from build123d import *

# Parameters (mm, degrees)
SKETCH2_R          = 32.5
CUT_EXTRUDE1_DEPTH = 3
SKETCH3_R          = 1.25
CUT_EXTRUDE2_DEPTH = 12
CUT_EXTRUDE3_REACH = 44.5
SKETCH4_R          = 1.25
SKETCH4_R_2        = 2.1
CHAMFER1_SIZE      = 0.5
CHAMFER2_SIZE      = 0.5


with BuildPart() as part:
    # Sketch1 → Revolve1 (revolve)
    with BuildSketch(Plane.YX):
        Polygon((-32.5, -4.5), (-32.5, -0.5), (-25, -0.5), (-25, 0), (-22.5, 0), (-22.5, 7), (-14, 7), (-14, 10.5), (-10.5, 10.5), (-10.5, 38), (-8.5, 38), (-8.5, 30), (0, 30), (0, 9.5), (-8, 9.5), (-8, 4.5), (-20, 4.5), (-20, -7.5), (-24, -7.5), (-24, -4.5), align=None)
    revolve(axis=Axis((0, 0, 0), (1, 0, 0)))

    # Sketch2 → Cut-Extrude1 (cut)
    with BuildSketch(Plane.ZY.offset(7.5)):
        Circle(SKETCH2_R)
        with BuildLine():
            Line((-8.94427191, 22), (8.94427191, 22))
            ThreePointArc((8.94427191, 22), (9.598925581, 21.927700219), (10.22202504, 21.714285714))
            ThreePointArc((10.22202504, 21.714285714), (16.970562748, 16.970562748), (21.714285714, 10.22202504))
            ThreePointArc((21.714285714, 10.22202504), (21.927700219, 9.598925581), (22, 8.94427191))
            Line((22, 8.94427191), (22, -8.94427191))
            ThreePointArc((22, -8.94427191), (21.927700219, -9.598925581), (21.714285714, -10.22202504))
            ThreePointArc((21.714285714, -10.22202504), (16.970562748, -16.970562748), (10.22202504, -21.714285714))
            ThreePointArc((10.22202504, -21.714285714), (9.598925581, -21.927700219), (8.94427191, -22))
            Line((8.94427191, -22), (-8.94427191, -22))
            ThreePointArc((-8.94427191, -22), (-9.598925581, -21.927700219), (-10.22202504, -21.714285714))
            ThreePointArc((-10.22202504, -21.714285714), (-16.970562748, -16.970562748), (-21.714285714, -10.22202504))
            ThreePointArc((-21.714285714, -10.22202504), (-21.927700219, -9.598925581), (-22, -8.94427191))
            Line((-22, -8.94427191), (-22, 8.94427191))
            ThreePointArc((-22, 8.94427191), (-21.927700219, 9.598925581), (-21.714285714, 10.22202504))
            ThreePointArc((-21.714285714, 10.22202504), (-16.970562748, 16.970562748), (-10.22202504, 21.714285714))
            ThreePointArc((-10.22202504, 21.714285714), (-9.598925581, 21.927700219), (-8.94427191, 22))
        make_face(mode=Mode.SUBTRACT)
    extrude(amount=-CUT_EXTRUDE1_DEPTH, mode=Mode.SUBTRACT)

    # Sketch3 → Cut-Extrude2 (cut)
    with BuildSketch(Plane(origin=(30, 0, 0), x_dir=(0, 0, -1), z_dir=(1, 0, 0))):
        with Locations((0, 6)):
            Circle(SKETCH3_R)
        with Locations((5.706339098, 1.854101966)):
            Circle(SKETCH3_R)
        with Locations((3.526711514, -4.854101966)):
            Circle(SKETCH3_R)
        with Locations((-3.526711514, -4.854101966)):
            Circle(SKETCH3_R)
        with Locations((-5.706339098, 1.854101966)):
            Circle(SKETCH3_R)
    extrude(amount=-CUT_EXTRUDE2_DEPTH, mode=Mode.SUBTRACT)

    # Sketch4 → Cut-Extrude3 (cut, up to next)
    with BuildSketch(Plane.ZY.offset(4.5), mode=Mode.PRIVATE) as cut_extrude3_sk1:
        with Locations((0, 27)):
            Circle(SKETCH4_R)
    cut_extrude3_tool1 = extrude(cut_extrude3_sk1.sketch, amount=-CUT_EXTRUDE3_REACH, mode=Mode.PRIVATE) & part.part
    add(cut_extrude3_tool1.solids().sort_by_distance((-4.5, 27, 0))[0], mode=Mode.SUBTRACT)
    # Sketch4 → Cut-Extrude3 (cut, up to next)
    with BuildSketch(Plane.ZY.offset(4.5), mode=Mode.PRIVATE) as cut_extrude3_sk2:
        with Locations((10.906477822, 26.330566677)):
            Circle(SKETCH4_R_2)
    cut_extrude3_tool2 = extrude(cut_extrude3_sk2.sketch, amount=-CUT_EXTRUDE3_REACH, mode=Mode.PRIVATE) & part.part
    add(cut_extrude3_tool2.solids().sort_by_distance((-4.5, 26.330567, 10.906478))[0], mode=Mode.SUBTRACT)
    # Sketch4 → Cut-Extrude3 (cut, up to next)
    with BuildSketch(Plane.ZY.offset(4.5), mode=Mode.PRIVATE) as cut_extrude3_sk3:
        with Locations((19.091883092, 19.091883092)):
            Circle(SKETCH4_R)
    cut_extrude3_tool3 = extrude(cut_extrude3_sk3.sketch, amount=-CUT_EXTRUDE3_REACH, mode=Mode.PRIVATE) & part.part
    add(cut_extrude3_tool3.solids().sort_by_distance((-4.5, 19.091883, 19.091883))[0], mode=Mode.SUBTRACT)
    # Sketch4 → Cut-Extrude3 (cut, up to next)
    with BuildSketch(Plane.ZY.offset(4.5), mode=Mode.PRIVATE) as cut_extrude3_sk4:
        with Locations((26.330566677, 10.906477822)):
            Circle(SKETCH4_R_2)
    cut_extrude3_tool4 = extrude(cut_extrude3_sk4.sketch, amount=-CUT_EXTRUDE3_REACH, mode=Mode.PRIVATE) & part.part
    add(cut_extrude3_tool4.solids().sort_by_distance((-4.5, 10.906478, 26.330567))[0], mode=Mode.SUBTRACT)
    # Sketch4 → Cut-Extrude3 (cut, up to next)
    with BuildSketch(Plane.ZY.offset(4.5), mode=Mode.PRIVATE) as cut_extrude3_sk5:
        with Locations((27, 0)):
            Circle(SKETCH4_R)
    cut_extrude3_tool5 = extrude(cut_extrude3_sk5.sketch, amount=-CUT_EXTRUDE3_REACH, mode=Mode.PRIVATE) & part.part
    add(cut_extrude3_tool5.solids().sort_by_distance((-4.5, 0, 27))[0], mode=Mode.SUBTRACT)
    # Sketch4 → Cut-Extrude3 (cut, up to next)
    with BuildSketch(Plane.ZY.offset(4.5), mode=Mode.PRIVATE) as cut_extrude3_sk6:
        with Locations((26.330566677, -10.906477822)):
            Circle(SKETCH4_R_2)
    cut_extrude3_tool6 = extrude(cut_extrude3_sk6.sketch, amount=-CUT_EXTRUDE3_REACH, mode=Mode.PRIVATE) & part.part
    add(cut_extrude3_tool6.solids().sort_by_distance((-4.5, -10.906478, 26.330567))[0], mode=Mode.SUBTRACT)
    # Sketch4 → Cut-Extrude3 (cut, up to next)
    with BuildSketch(Plane.ZY.offset(4.5), mode=Mode.PRIVATE) as cut_extrude3_sk7:
        with Locations((19.091883092, -19.091883092)):
            Circle(SKETCH4_R)
    cut_extrude3_tool7 = extrude(cut_extrude3_sk7.sketch, amount=-CUT_EXTRUDE3_REACH, mode=Mode.PRIVATE) & part.part
    add(cut_extrude3_tool7.solids().sort_by_distance((-4.5, -19.091883, 19.091883))[0], mode=Mode.SUBTRACT)
    # Sketch4 → Cut-Extrude3 (cut, up to next)
    with BuildSketch(Plane.ZY.offset(4.5), mode=Mode.PRIVATE) as cut_extrude3_sk8:
        with Locations((10.906477822, -26.330566677)):
            Circle(SKETCH4_R_2)
    cut_extrude3_tool8 = extrude(cut_extrude3_sk8.sketch, amount=-CUT_EXTRUDE3_REACH, mode=Mode.PRIVATE) & part.part
    add(cut_extrude3_tool8.solids().sort_by_distance((-4.5, -26.330567, 10.906478))[0], mode=Mode.SUBTRACT)
    # Sketch4 → Cut-Extrude3 (cut, up to next)
    with BuildSketch(Plane.ZY.offset(4.5), mode=Mode.PRIVATE) as cut_extrude3_sk9:
        with Locations((0, -27)):
            Circle(SKETCH4_R)
    cut_extrude3_tool9 = extrude(cut_extrude3_sk9.sketch, amount=-CUT_EXTRUDE3_REACH, mode=Mode.PRIVATE) & part.part
    add(cut_extrude3_tool9.solids().sort_by_distance((-4.5, -27, 0))[0], mode=Mode.SUBTRACT)
    # Sketch4 → Cut-Extrude3 (cut, up to next)
    with BuildSketch(Plane.ZY.offset(4.5), mode=Mode.PRIVATE) as cut_extrude3_sk10:
        with Locations((-10.906477822, -26.330566677)):
            Circle(SKETCH4_R_2)
    cut_extrude3_tool10 = extrude(cut_extrude3_sk10.sketch, amount=-CUT_EXTRUDE3_REACH, mode=Mode.PRIVATE) & part.part
    add(cut_extrude3_tool10.solids().sort_by_distance((-4.5, -26.330567, -10.906478))[0], mode=Mode.SUBTRACT)
    # Sketch4 → Cut-Extrude3 (cut, up to next)
    with BuildSketch(Plane.ZY.offset(4.5), mode=Mode.PRIVATE) as cut_extrude3_sk11:
        with Locations((-19.091883092, -19.091883092)):
            Circle(SKETCH4_R)
    cut_extrude3_tool11 = extrude(cut_extrude3_sk11.sketch, amount=-CUT_EXTRUDE3_REACH, mode=Mode.PRIVATE) & part.part
    add(cut_extrude3_tool11.solids().sort_by_distance((-4.5, -19.091883, -19.091883))[0], mode=Mode.SUBTRACT)
    # Sketch4 → Cut-Extrude3 (cut, up to next)
    with BuildSketch(Plane.ZY.offset(4.5), mode=Mode.PRIVATE) as cut_extrude3_sk12:
        with Locations((-26.330566677, -10.906477822)):
            Circle(SKETCH4_R_2)
    cut_extrude3_tool12 = extrude(cut_extrude3_sk12.sketch, amount=-CUT_EXTRUDE3_REACH, mode=Mode.PRIVATE) & part.part
    add(cut_extrude3_tool12.solids().sort_by_distance((-4.5, -10.906478, -26.330567))[0], mode=Mode.SUBTRACT)
    # Sketch4 → Cut-Extrude3 (cut, up to next)
    with BuildSketch(Plane.ZY.offset(4.5), mode=Mode.PRIVATE) as cut_extrude3_sk13:
        with Locations((-27, 0)):
            Circle(SKETCH4_R)
    cut_extrude3_tool13 = extrude(cut_extrude3_sk13.sketch, amount=-CUT_EXTRUDE3_REACH, mode=Mode.PRIVATE) & part.part
    add(cut_extrude3_tool13.solids().sort_by_distance((-4.5, 0, -27))[0], mode=Mode.SUBTRACT)
    # Sketch4 → Cut-Extrude3 (cut, up to next)
    with BuildSketch(Plane.ZY.offset(4.5), mode=Mode.PRIVATE) as cut_extrude3_sk14:
        with Locations((-26.330566677, 10.906477822)):
            Circle(SKETCH4_R_2)
    cut_extrude3_tool14 = extrude(cut_extrude3_sk14.sketch, amount=-CUT_EXTRUDE3_REACH, mode=Mode.PRIVATE) & part.part
    add(cut_extrude3_tool14.solids().sort_by_distance((-4.5, 10.906478, -26.330567))[0], mode=Mode.SUBTRACT)
    # Sketch4 → Cut-Extrude3 (cut, up to next)
    with BuildSketch(Plane.ZY.offset(4.5), mode=Mode.PRIVATE) as cut_extrude3_sk15:
        with Locations((-19.091883092, 19.091883092)):
            Circle(SKETCH4_R)
    cut_extrude3_tool15 = extrude(cut_extrude3_sk15.sketch, amount=-CUT_EXTRUDE3_REACH, mode=Mode.PRIVATE) & part.part
    add(cut_extrude3_tool15.solids().sort_by_distance((-4.5, 19.091883, -19.091883))[0], mode=Mode.SUBTRACT)
    # Sketch4 → Cut-Extrude3 (cut, up to next)
    with BuildSketch(Plane.ZY.offset(4.5), mode=Mode.PRIVATE) as cut_extrude3_sk16:
        with Locations((-10.906477822, 26.330566677)):
            Circle(SKETCH4_R_2)
    cut_extrude3_tool16 = extrude(cut_extrude3_sk16.sketch, amount=-CUT_EXTRUDE3_REACH, mode=Mode.PRIVATE) & part.part
    add(cut_extrude3_tool16.solids().sort_by_distance((-4.5, 26.330567, -10.906478))[0], mode=Mode.SUBTRACT)

    # Chamfer1
    chamfer1_edges = [part.edges().sort_by_distance(p)[0] for p in [
        (-7.5, 16.970562748, 16.970562748),
        (-7.5, 20, 0),
        (-7.5, 16.970562748, -16.970562748),
        (-7.5, -16.970562748, -16.970562748),
        (-7.5, -16.970562748, 16.970562748),
        (-7.5, -9.598925581, 21.927700219),
        (-7.5, -21.927700219, 9.598925581),
        (-7.5, -22, 0),
        (-7.5, -21.927700219, -9.598925581),
        (-7.5, -9.598925581, -21.927700219),
        (-7.5, 0, -22),
        (-7.5, 9.598925581, -21.927700219),
        (-7.5, 21.927700219, -9.598925581),
        (-7.5, 22, 0),
        (-7.5, 21.927700219, 9.598925581),
        (-7.5, 9.598925581, 21.927700219),
        (-7.5, 0, 22),
    ]]
    chamfer(chamfer1_edges, length=CHAMFER1_SIZE)

    # Chamfer2
    chamfer2_edges = [part.edges().sort_by_distance(p)[0] for p in [
        (-4.5, 32.5, 0),
    ]]
    chamfer(chamfer2_edges, length=CHAMFER2_SIZE)


solid = part.part
Can you work these out from the model? Positions are in its coordinate system, mm. A direction names the side the tool comes from. Give positions to 0.01 mm unless a question says otherwise; leave off trailing zeros. Order: outer loops, then holes, each group sorted by start corner. A loop starts at its lowest first (then second) coordinate and runs counter-clockwise, first axis right, second up. Notation, with made-up numbers: M 47,-32.5 L 84,-32.5 A20 cw 84,-6.5 Z; hole C 49,81 d11. An arc over 180 degrees is marked long. One line per question, with ' | ' between items.
Item 1: We'd pull the mould along Y, two halves only. Please class faces 1 (the face through (6.96, 1.73, 7.81)), 2 (the face through (-5.77, 17.05, 16.89)), 3 (the face through (0, 22.34, -3.82)): released by +Y, released by -Y, zero draft, split by the parting line, or undercut.
Answer block:
face 1: undercut | face 2: released by +Y | face 3: zero draft
Item 2: Suppose I cut it at C-C, the plane x = 17. Write out the boundary of the cut face in (y, z).
Answer block:
outline: C 0,0 d21
Item 3: For faces 4 (the face through (-5.77, -16.89, 17.05)), 5 (the face through (-1.33, 4.336, 19.524)), 6 (the face through (7, 10.32, 9.69)), 7 (the face through (-5.77, -17.05, -16.89)), 8 (the face through (-5.77, 16.89, -17.05)), which set-ups out of +Z, -Z, +X, -X, +Y, -Y let a thin tool reach every point of the face, with its end or its side?
Answer block:
face 4: +Z, -X, -Y | face 5: -X | face 6: +X | face 7: -Z, -X, -Y | face 8: -Z, -X, +Y
Item 4: Suppose I cut it at A-A, the plane x = -3. Give the number of separate pieces and of enclosed holes in the cut face, then the cut area to 3 significant figures.
Answer block:
separate pieces: 1 | enclosed holes: 17 | area: 1,910 mm2
Item 5: I'm going to push flat-ended pins straight in: pin 1 Ø1.2 at (y, z) = (-5.5, -3) entering from +X; pin 2 Ø15.5 at (y, z) = (0, 0) entering from -X; pin 3 Ø3 at (y, z) = (0, 27) entering from +X. Where does each tip first touch, or does it pass through?
Answer block:
pin 1: stops at x = 30 | pin 2: stops at x = 9.5 | pin 3: stops at x = -0.5
Item 6: Please list where these lines run through material, in increasing order: L1, parallel to Y at x = -2.1, z = -27; L2, parallel to X at y = 17.5, z = 20.5; L3, parallel to X at y = -15.5, z = 3.
Answer block:
L1: y = -18.09 to -12.9, -8.92 to -1.25, 1.25 to 8.92, 12.9 to 18.09 | L2: x = -4.5 to -0.5 | L3: x = 4.5 to 7
Item 7: Suppose I cut it at B-B, the plane x = 24. Write out the boundary of the cut face in (y, z), then the cut area to 3 significant figures.
Answer block:
outline: C 0,0 d21; hole C -4.85,-3.53 d2.5; hole C -4.85,3.53 d2.5; hole C 1.85,-5.71 d2.5; hole C 1.85,5.71 d2.5; hole C 6,0 d2.5 | area: 322 mm2
